CAD build for the part. Positions are in the model's coordinates, mm. A direction names the side the tool comes from. Coordinates: 2 decimals unless noted, no trailing zeros. Loops run counter-clockwise (first coordinate to the right, second up) from the corner with the lowest first, then second, coordinate; pieces in that order, holes last. Notation, with made-up numbers: (-39, 11.25) -> (-12, 11.25) arc R15 cw to (-12, 35.25) -> close; hole circle Ø4 at (-25.5, -2.5). An arc over 180 degrees is marked (long way). Return JSON: item names as keys, results as strings. Group by question number.
(1) Saw through at C-C on y = 1. Give the number of separate pieces and of enclosed holes in the cut face, then the cut area to 3 significant figures.
(2) Saw through at A-A on z = 0. Write the cut outline in (x, y).
(3) Probe L1, parallel to Z at x = 0, y = 1.05 (3 decimals); L2, parallel to X at y = 1.45, z = -31.5; L3, parallel to X at y = 0.4, z = -4. List the from-to ranges inside material, lowest first.
(4) Saw through at B-B on x = 0. Write the cut outline in (y, z) (3 decimals), then the cut area to 3 significant figures.
(5) Flat gauge pins, fed straight in: pin 1 Ø0.7 at (y, z) = (1, -3.5) entering from -X; pin 2 Ø12 at (x, z) = (-31.82, 31.82) entering from +Y; pin 3 Ø0.5 at (x, y) = (-11.5, 1) entering from +Z (3 decimals); pin 4 Ø0.5 at (x, y) = (-6.5, 1.5) entering from -Z (3 decimals). Where does each tip first touch, or does it go through?
(6) Tool access for faces 4 (the face through (-9, 1, 11.875)), 5 (the face through (-25.506, 0.863, -14.3)), 6 (the face through (16.265, 1, 3)): list every direction of +Z, -Z, +X, -X, +Y, -Y with a clear straight run to the whole face (end or side of a thin tool).
(7) Mould opens along Z. For faces 1 (the face through (0, 1.75, 0)), 2 (the face through (-16.265, 1, 3)), 3 (the face through (-9, 1, -11.875)) say: pulls with the +Z half, pulls with the -Z half, needs draft (parallel to the pull), parting line crosses it, or undercut.
```python
from build123d import *

# Parameters (mm, degrees)
SKETCH1_R           = 5.125
BOSS_EXTRUDE1_DEPTH = 1.75
CUT_EXTRUDE2_REACH  = 3.75
FILLET1_R           = 1
SKETCH4_R           = 2.5
SKETCH4_R_2         = 1
BOSS_EXTRUDE2_DEPTH = 1.75
FILLET2_R           = 1


with BuildPart() as part:
    # Sketch1 → Boss-Extrude1 (new body)
    with BuildSketch(Plane(origin=(0, 0, 0), x_dir=(1, 0, 0), z_dir=(0, 1, 0))):
        with BuildLine():
            Line((19.25, -4.372796114), (19.25, 4.372796114))
            Line((19.25, 4.372796114), (31.727014355, 24.170367928))
            ThreePointArc((31.727014355, 24.170367928), (35.898606592, 38.291735223), (24.95898291, 28.435781196))
            Line((24.95898291, 28.435781196), (14.52188958, 11.875))
            Line((14.52188958, 11.875), (-14.52188958, 11.875))
            Line((-14.52188958, 11.875), (-24.95898291, 28.435781196))
            ThreePointArc((-24.95898291, 28.435781196), (-35.898606592, 38.291735223), (-31.727014355, 24.170367928))
            Line((-31.727014355, 24.170367928), (-19.25, 4.372796114))
            Line((-19.25, 4.372796114), (-19.25, -4.372796114))
            Line((-19.25, -4.372796114), (-31.727014355, -24.170367928))
            ThreePointArc((-31.727014355, -24.170367928), (-35.898606592, -38.291735223), (-24.95898291, -28.435781196))
            Line((-24.95898291, -28.435781196), (-14.52188958, -11.875))
            Line((-14.52188958, -11.875), (14.52188958, -11.875))
            Line((14.52188958, -11.875), (24.95898291, -28.435781196))
            ThreePointArc((24.95898291, -28.435781196), (35.898606592, -38.291735223), (31.727014355, -24.170367928))
            Line((31.727014355, -24.170367928), (19.25, -4.372796114))
        make_face()
        with Locations((-31.819805153, 31.819805153)):
            Circle(SKETCH1_R, mode=Mode.SUBTRACT)
        with Locations((31.819805153, 31.819805153)):
            Circle(SKETCH1_R, mode=Mode.SUBTRACT)
        with Locations((-31.819805153, -31.819805153)):
            Circle(SKETCH1_R, mode=Mode.SUBTRACT)
        with Locations((31.819805153, -31.819805153)):
            Circle(SKETCH1_R, mode=Mode.SUBTRACT)
    extrude(amount=BOSS_EXTRUDE1_DEPTH)

    # Sketch2 → Cut-Extrude2 (cut, up to next)
    with BuildSketch(Plane(origin=(0, 1.75, 0), x_dir=(1, 0, 0), z_dir=(0, 1, 0)), mode=Mode.PRIVATE) as cut_extrude2_sk1:
        with BuildLine():
            ThreePointArc((-27.955034886, 28.453921053), (-29.087274778, 27.484035009), (-30.450746481, 26.88104991))
            Line((-30.450746481, 26.88104991), (-16.265380297, 4.372796114))
            Line((-16.265380297, 4.372796114), (-16.265380297, 1.2625))
            Line((-16.265380297, 1.2625), (-1.2625, 1.2625))
            Line((-1.2625, 1.2625), (-1.2625, 9.35))
            Line((-1.2625, 9.35), (-15.915179722, 9.35))
            Line((-15.915179722, 9.35), (-27.955034886, 28.453921053))
        make_face()
    cut_extrude2_tool1 = extrude(cut_extrude2_sk1.sketch, amount=-CUT_EXTRUDE2_REACH, mode=Mode.PRIVATE) & part.part
    add(cut_extrude2_tool1.solids().sort_by_distance((-22.27259, 1.75, -18.689269))[0], mode=Mode.SUBTRACT)
    # Sketch2 → Cut-Extrude2 (cut, up to next)
    with BuildSketch(Plane(origin=(0, 1.75, 0), x_dir=(1, 0, 0), z_dir=(0, 1, 0)), mode=Mode.PRIVATE) as cut_extrude2_sk2:
        with BuildLine():
            Line((-16.265380297, -1.2625), (-16.265380297, -4.372796114))
            Line((-16.265380297, -4.372796114), (-30.450746481, -26.88104991))
            ThreePointArc((-30.450746481, -26.88104991), (-29.087274778, -27.484035009), (-27.955034886, -28.453921053))
            Line((-27.955034886, -28.453921053), (-15.915179722, -9.35))
            Line((-15.915179722, -9.35), (-1.2625, -9.35))
            Line((-1.2625, -9.35), (-1.2625, -1.2625))
            Line((-1.2625, -1.2625), (-16.265380297, -1.2625))
        make_face()
    cut_extrude2_tool2 = extrude(cut_extrude2_sk2.sketch, amount=-CUT_EXTRUDE2_REACH, mode=Mode.PRIVATE) & part.part
    add(cut_extrude2_tool2.solids().sort_by_distance((-15.866466, 1.75, 2.817648))[0], mode=Mode.SUBTRACT)
    # Sketch2 → Cut-Extrude2 (cut, up to next)
    with BuildSketch(Plane(origin=(0, 1.75, 0), x_dir=(1, 0, 0), z_dir=(0, 1, 0)), mode=Mode.PRIVATE) as cut_extrude2_sk3:
        with BuildLine():
            Line((15.915179722, 9.35), (1.2625, 9.35))
            Line((1.2625, 9.35), (1.2625, 1.2625))
            Line((1.2625, 1.2625), (16.265380297, 1.2625))
            Line((16.265380297, 1.2625), (16.265380297, 4.372796114))
            Line((16.265380297, 4.372796114), (30.450746481, 26.88104991))
            ThreePointArc((30.450746481, 26.88104991), (29.087274778, 27.484035009), (27.955034886, 28.453921053))
            Line((27.955034886, 28.453921053), (15.915179722, 9.35))
        make_face()
    cut_extrude2_tool3 = extrude(cut_extrude2_sk3.sketch, amount=-CUT_EXTRUDE2_REACH, mode=Mode.PRIVATE) & part.part
    add(cut_extrude2_tool3.solids().sort_by_distance((22.27259, 1.75, -18.689269))[0], mode=Mode.SUBTRACT)
    # Sketch2 → Cut-Extrude2 (cut, up to next)
    with BuildSketch(Plane(origin=(0, 1.75, 0), x_dir=(1, 0, 0), z_dir=(0, 1, 0)), mode=Mode.PRIVATE) as cut_extrude2_sk4:
        with BuildLine():
            Line((1.2625, -1.2625), (1.2625, -9.35))
            Line((1.2625, -9.35), (15.915179722, -9.35))
            Line((15.915179722, -9.35), (27.955034886, -28.453921053))
            ThreePointArc((27.955034886, -28.453921053), (29.087274778, -27.484035009), (30.450746481, -26.88104991))
            Line((30.450746481, -26.88104991), (16.265380297, -4.372796114))
            Line((16.265380297, -4.372796114), (16.265380297, -1.2625))
            Line((16.265380297, -1.2625), (1.2625, -1.2625))
        make_face()
    cut_extrude2_tool4 = extrude(cut_extrude2_sk4.sketch, amount=-CUT_EXTRUDE2_REACH, mode=Mode.PRIVATE) & part.part
    add(cut_extrude2_tool4.solids().sort_by_distance((28.874583, 1.75, 27.146552))[0], mode=Mode.SUBTRACT)

    # Fillet1
    fillet1_edges = [part.edges().sort_by_distance(p)[0] for p in [
        (16.265380297, 0.875, -1.2625),
        (1.2625, 0.875, -1.2625),
        (1.2625, 0.875, -9.35),
        (15.915179722, 0.875, -9.35),
        (27.955034886, 0.875, -28.453921053),
        (30.450746481, 0.875, -26.88104991),
        (16.265380297, 0.875, -4.372796114),
        (-31.727014355, 0.875, 24.170367928),
        (-19.25, 0.875, 4.372796114),
        (-14.52188958, 0.875, 11.875),
        (-24.95898291, 0.875, 28.435781196),
        (1.2625, 0.875, 1.2625),
        (16.265380297, 0.875, 1.2625),
        (16.265380297, 0.875, 4.372796114),
        (30.450746481, 0.875, 26.88104991),
        (27.955034886, 0.875, 28.453921053),
        (15.915179722, 0.875, 9.35),
        (1.2625, 0.875, 9.35),
        (-16.265380297, 0.875, 1.2625),
        (-1.2625, 0.875, 1.2625),
        (-15.915179722, 0.875, 9.35),
        (-27.955034886, 0.875, 28.453921053),
        (-30.450746481, 0.875, 26.88104991),
        (-16.265380297, 0.875, 4.372796114),
        (-31.727014355, 0.875, -24.170367928),
        (-19.25, 0.875, -4.372796114),
        (-14.52188958, 0.875, -11.875),
        (-24.95898291, 0.875, -28.435781196),
        (31.727014355, 0.875, 24.170367928),
        (19.25, 0.875, 4.372796114),
        (14.52188958, 0.875, 11.875),
        (24.95898291, 0.875, 28.435781196),
        (24.95898291, 0.875, -28.435781196),
        (14.52188958, 0.875, -11.875),
        (19.25, 0.875, -4.372796114),
        (31.727014355, 0.875, -24.170367928),
        (-1.2625, 0.875, -1.2625),
        (-16.265380297, 0.875, -1.2625),
        (-16.265380297, 0.875, -4.372796114),
        (-30.450746481, 0.875, -26.88104991),
        (-27.955034886, 0.875, -28.453921053),
        (-15.915179722, 0.875, -9.35),
        (-1.2625, 0.875, -9.35),
    ]]
    fillet(fillet1_edges, radius=FILLET1_R)

    # Sketch4 → Boss-Extrude2 (add)
    with BuildSketch(Plane.XZ):
        with Locations((-20.75, 0)):
            Circle(SKETCH4_R)
        with Locations((-20.75, 0)):
            Circle(SKETCH4_R_2, mode=Mode.SUBTRACT)
        with Locations((0, -13.375)):
            Circle(SKETCH4_R)
        Polygon((0.866025404, -11.875), (-0.866025404, -11.875), (-1.732050808, -13.375), (-0.866025404, -14.875), (0.866025404, -14.875), (1.732050808, -13.375), align=None, mode=Mode.SUBTRACT)
        Polygon((1.732050808, -13.375), (0.866025404, -11.875), (-0.866025404, -11.875), (-1.732050808, -13.375), (-0.866025404, -14.875), (0.866025404, -14.875), align=None)
        with Locations((0, -13.375)):
            Circle(SKETCH4_R_2, mode=Mode.SUBTRACT)
        with Locations((0, 13.375)):
            Circle(SKETCH4_R)
        with Locations((0, 13.375)):
            Circle(SKETCH4_R_2, mode=Mode.SUBTRACT)
    extrude(amount=-BOSS_EXTRUDE2_DEPTH)

    # Fillet2
    fillet2_edges = [part.edges().sort_by_distance(p)[0] for p in [
        (-19.25, 0.875, -2),
        (-19.25, 0.875, 2),
        (-2, 0.875, -11.875),
        (2, 0.875, -11.875),
        (-2, 0.875, 11.875),
        (2, 0.875, 11.875),
    ]]
    fillet(fillet2_edges, radius=FILLET2_R)


solid = part.part
```
Geometry results:
{
 "1": {"separate pieces": "1", "enclosed holes": "7", "area": "1,190 mm²"},
 "2": {"outline": "(-23.25, 0) -> (-21.75, 0) -> (-21.75, 1.75) -> (-23.25, 1.75) -> close; (-19.75, 0) -> (19.25, 0) -> (19.25, 1.75) -> (-19.75, 1.75) -> close"},
 "3": {"L1": "-15.875 to -14.375, -12.375 to 12.375, 14.375 to 15.875", "L2": "-39.46 to -36.93, -26.7 to -24.18, 24.18 to 26.7, 36.93 to 39.46", "L3": "-19.25 to -16.27, -1.26 to 1.26, 16.27 to 19.25"},
 "4": {"outline": "(0, -15.875) -> (1.75, -15.875) -> (1.75, -14.375) -> (0, -14.375) -> close; (0, -12.375) -> (1.75, -12.375) -> (1.75, 12.375) -> (0, 12.375) -> close; (0, 14.375) -> (1.75, 14.375) -> (1.75, 15.875) -> (0, 15.875) -> close", "area": "48.6 mm²"},
 "5": {"pin 1": "x = -19.3", "pin 2": "y = 1.75", "pin 3": "z = 11.875", "pin 4": "z = -11.875"},
 "6": {"face 4": "+Z, +Y, -Y", "face 5": "-X, +Y, -Y", "face 6": "+Y, -Y"},
 "7": {"face 1": "needs draft", "face 2": "undercut", "face 3": "pulls with the -Z half"}
}
